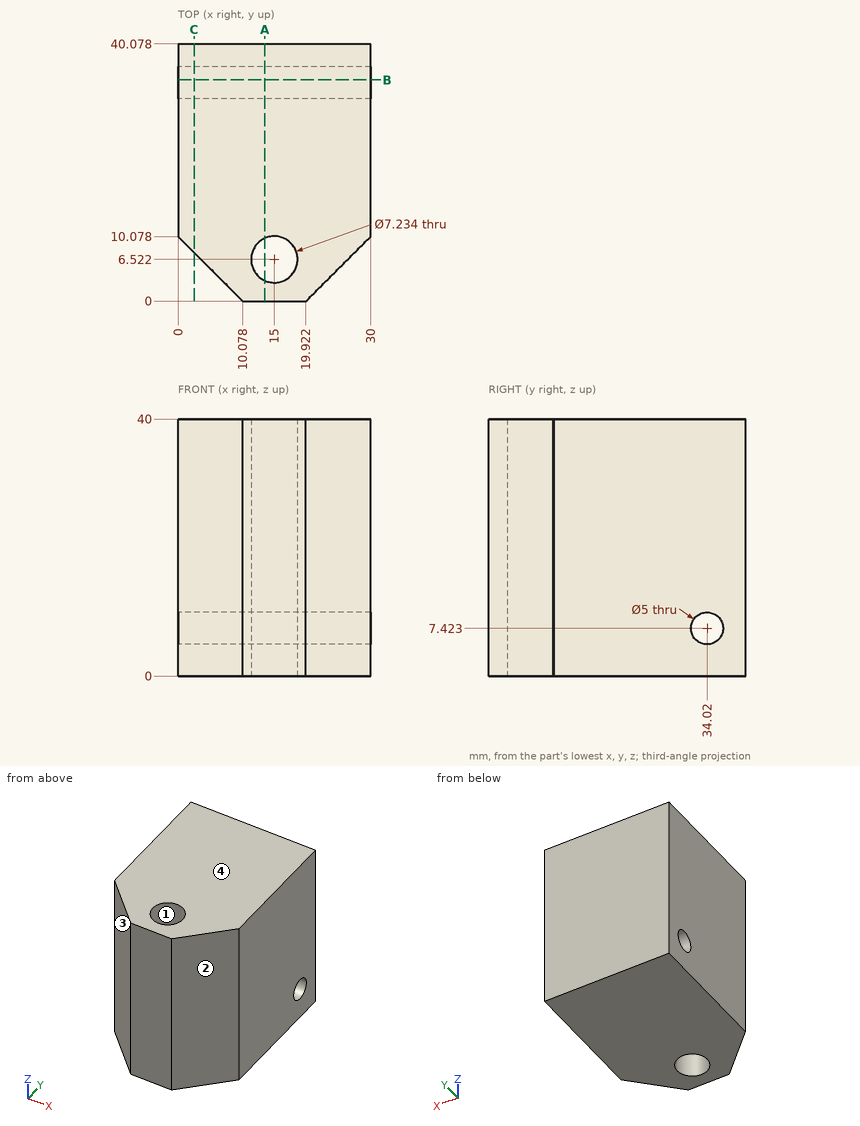
Design review of the part shown in the three views and the two pictorial views. Dimensions are in mm from the part's minimum x, y and z. Give positions to 0.01 mm unless a question says otherwise; leave off trailing zeros. Loops run counter-clockwise (first coordinate to the right, second up) from the corner with the lowest first, then second, coordinate; pieces in that order, holes last. Notation, with made-up numbers: M 77.25,62.5 L 93.25,62.5 A7 cw 93.25,68.5 Z; hole C 46,-31 d1. An arc over 180 degrees is marked long. Answer as a JSON object with one key per item and string values.
Item 1: For P1, Ø6, axis at x = 15, y = 6.52, coming from the +Z side, flat-tipped, find the tip position at first contact; note if it passes through.
Output values:
{"P1": "passes through"}
Item 2: We need section B-B (y = 34.5). State the section outline as (x, z) points.
Output values:
{"outline": "M 0,0 L 30,0 L 30,4.97 L 0,4.97 Z; M 0,9.88 L 30,9.88 L 30,40 L 0,40 Z"}
Item 3: Mouldability with a two-part tool opening along X and no side actions: class the marked faces 1, 2, 3 and 4 as pulls with the +X half, pulls with the -X half, needs draft (parallel to the pull), parting line crosses it, or undercut.
Output values:
{"face 1": "undercut", "face 2": "pulls with the +X half", "face 3": "pulls with the -X half", "face 4": "needs draft"}
Item 4: We need section C-C (x = 2.5). State the section outline as (y, z) points, and give its area (3 significant figures).
Output values:
{"outline": "M 7.58,0 L 40.08,0 L 40.08,40 L 7.58,40 Z; hole C 34.02,7.42 d5", "area": "1,280 mm2"}
Item 5: Wall thickness on line 1 along Y through (x, z) = (15, 17.5) (1 decimal); line 2 along Z through (x, y) = (2.5, 34); line 3 along Y through (x, z) = (13.75, 17.5) (1 decimal): over which ranges is each line inside the solid? List them lowest first.
Output values:
{"line 1": "y = 0 to 2.9, 10.1 to 40.1", "line 2": "z = 0 to 4.92, 9.92 to 40", "line 3": "y = 0 to 3.1, 9.9 to 40.1"}
Item 6: We need section A-A (x = 13.5). State the section outline as (y, z) points.
Output values:
{"outline": "M 0,0 L 3.23,0 L 3.23,40 L 0,40 Z; M 9.81,0 L 40.08,0 L 40.08,40 L 9.81,40 Z; hole C 34.02,7.42 d5"}
